from build123d import *

# Parameters (mm, degrees)
SKETCH1_R           = 6.35
BOSS_EXTRUDE1_DEPTH = 2.54
BOSS_EXTRUDE2_DEPTH = 3.175
SKETCH3_R           = 1.27
CUT_EXTRUDE7_DEPTH  = 158.509352305


with BuildPart() as part:
    # Sketch1 → Boss-Extrude1 (new body)
    with BuildSketch(Plane(origin=(0, 0, 0), x_dir=(1, 0, 0), z_dir=(0, 1, 0))):
        with Locations(Location((0, 0, 0), (0, 0, 270))):
            Circle(SKETCH1_R)
    extrude(amount=BOSS_EXTRUDE1_DEPTH)

    # Sketch2 → Boss-Extrude2 (add, symmetric)
    with BuildSketch(Plane(origin=(0, 0, 0), x_dir=(0, 0, -1), z_dir=(1, 0, 0))):
        Polygon((105.518009423, 112.548137483), (110.008137483, 108.058009423), (4.490128061, 2.54), (0, 2.54), (0, 7.030128061), align=None)
    extrude(amount=BOSS_EXTRUDE2_DEPTH, both=True)

    # Sketch3 → Cut-Extrude7 (cut, through all)
    with BuildSketch(Plane.XZ):
        with Locations(Location((0, 0, 0), (0, 0, 270))):
            Circle(SKETCH3_R)
    extrude(amount=-CUT_EXTRUDE7_DEPTH, mode=Mode.SUBTRACT)

    # Sketch2_4 → Revolve3 (revolve)
    with BuildSketch(Plane(origin=(0, 0, 0), x_dir=(0, 0, -1), z_dir=(1, 0, 0))):
        Polygon((105.518009423, 112.548137483), (110.008137483, 108.058009423), (4.490128061, 2.54), (0, 2.54), (0, 7.030128061), align=None)
    revolve(axis=Axis((0, 2.54, 0), (0, -1, 0)))


solid = part.part
For this review, take the finished solid that the model builds, in its own axes (mm). A direction names the side the tool comes from. Give positions to 0.01 mm unless a question says otherwise; leave off trailing zeros. Loops run counter-clockwise (first coordinate to the right, second up) from the corner with the lowest first, then second, coordinate; pieces in that order, holes last. Notation, with made-up numbers: (62.25, 23.5) - (99.25, 23.5) arc R36 ccw to (99.25, 62.5) - close; hole circle Ø8 at (-12, 12.25). An arc over 180 degrees is marked (long way). Write each question's results on one line, items separated by ' | '.
(1) Draft analysis for pull direction Y (two halves, no side actions). For faces 3 (the flat face through (2, 0, 0)), 4 (the conical face through (-103.28, 112.27, 22.94)), 5 (the flat face through (4, 2.54, 3)), state which applies: +Y half, -Y half, draft (parallel to the pull), parting line (faces both ways), or undercut.
Conclusion:
face 3: -Y half | face 4: +Y half | face 5: undercut
(2) For faces 1 (the cylindrical face through (-3.86, 1.25, -5.04)), 2 (the conical face through (9.03, 37.08, -28.66)), list the 3-axis set-ups (+Z, -Z, +X, -X, +Y, -Y) from which the entire face can be reached by the end or side of a thin tool; tool diameter is ignored.
Conclusion:
face 1: -Y | face 2: +Y
(3) Take a section at A-A (y = 81). Give the boundary of the cut face in (x, z) (3 decimals), then the cut area to 3 significant figures.
Conclusion:
outline: (-3.175, -82.95) - (3.175, -82.95) - (3.175, -82.889) arc R82.95 ccw (long way) to (-3.175, -82.889) - close; hole circle Ø147.94 at (0, 0) | area: 4,430 mm^2
(4) For pin 1 Ø5 at (x, y) = (42, 80.5) entering from +Z; pin 2 Ø1 at (y, z) = (43.5, 16.5) entering from -X; pin 3 Ø8 at (x, z) = (33.5, 17) entering from +Y, all flat-tipped, find the tip position at first contact; note any pin that passes through.
Conclusion:
pin 1: z = 74.17 | pin 2: x = -42.92 | pin 3: y = 48.6
(5) Take a section at B-B (y = 98). Give the boundary of the cut face in (x, z) (3 decimals).
Conclusion:
outline: (-3.175, -99.95) - (3.175, -99.95) - (3.175, -99.9) arc R99.95 ccw (long way) to (-3.175, -99.9) - close; hole circle Ø181.94 at (0, 0)
(6) For line 1 along X through (y, z) = (1, 0); line 2 along Z through (x, y) = (-40, 91.5); line 3 along X through (y, z) = (104.5, -3), list the stretches that pass through material, from the lowest coordinate up.
Conclusion:
line 1: -6.35 to -1.27, 1.27 to 6.35 | line 2: -84.46 to -74.4, 74.4 to 84.46 | line 3: -106.41 to -97.42, 97.42 to 106.41
